Part model, mm, in its own coordinate system. Round coordinates to 2 decimals unless told otherwise and drop trailing zeros. Write each loop counter-clockwise with the first axis right and the second up, starting at its lowest first coordinate (ties: lowest second). Pieces come first, ordered by that corner, then holes.
1) Saw through at A-A on x = 129. Write the cut outline in (y, z), and give its area (3 significant figures).
2) Drill centre lines: L1, parallel to X at y = -22, z = 7; L2, parallel to X at y = 15, z = 6; L3, parallel to Y at x = 233.5, z = 3.5. Where is each one in solid material? Low to high.
3) Flat gauge pins, fed straight in: pin 1 (16 mm diameter, centred on x = 60.5, z = 14, fed in from +Y); pin 2 (5 mm diameter, centred on x = 95, y = -11, fed in from -Z); pin 3 (2.5 mm diameter, centred on x = -59.5, z = 6.5, fed in from -Y). Where does each tip first touch, or does it go through?
```python
from build123d import *

# Parameters (mm, degrees)
SKETCH1_R           = 10
BOSS_EXTRUDE1_DEPTH = 20
BOSS_EXTRUDE2_DEPTH = 20
SKETCH5_R           = 20
BOSS_EXTRUDE3_DEPTH = 5
CUT_EXTRUDE2_DEPTH  = 20
BOSS_EXTRUDE4_DEPTH = 20
CUT_EXTRUDE9_DEPTH  = 20
SKETCH13_R          = 10
CUT_EXTRUDE10_DEPTH = 20


with BuildPart() as part:
    # Sketch1 → Boss-Extrude1 (new body)
    with BuildSketch(Plane.XY):
        with BuildLine():
            Line((-71.370560529, 20), (333.629439471, 20))
            ThreePointArc((333.629439471, 20), (353.629439471, 0), (333.629439471, -20))
            Line((333.629439471, -20), (-71.370560529, -20))
            ThreePointArc((-71.370560529, -20), (-91.370560529, 0), (-71.370560529, 20))
        make_face()
        with Locations((-71.370560529, 0)):
            Circle(SKETCH1_R, mode=Mode.SUBTRACT)
        with Locations((333.629439471, 0)):
            Circle(SKETCH1_R, mode=Mode.SUBTRACT)
    extrude(amount=BOSS_EXTRUDE1_DEPTH)

    # Sketch2 → Boss-Extrude2 (add)
    with BuildSketch(Plane(origin=(0, 0, 0), x_dir=(-1, 0, 0), z_dir=(0, 0, -1))):
        with BuildLine():
            Line((71.370560529, -20), (71.370560529, -25))
            ThreePointArc((71.370560529, -25), (64.900084402, -24.148145657), (58.870560529, -21.650635095))
            Line((58.870560529, -21.650635095), (62.564306071, -17.956889553))
            ThreePointArc((62.564306071, -17.956889553), (66.850482602, -19.482527955), (71.370560529, -20))
        make_face()
    boss_extrude2 = extrude(amount=BOSS_EXTRUDE2_DEPTH)

    # Sketch5 → Boss-Extrude3 (add)
    with BuildSketch(Plane.XY.offset(15)):
        with Locations((-72.002203934, 0)):
            Circle(SKETCH5_R)
    extrude(amount=BOSS_EXTRUDE3_DEPTH)

    # Mirror1: Boss-Extrude2 across plane
    add(boss_extrude2.mirror(Plane.ZX))

    # Sketch7 → Cut-Extrude2 (cut)
    with BuildSketch(Plane(origin=(0, 0, -20), x_dir=(-1, 0, 0), z_dir=(0, 0, -1))):
        with BuildLine():
            Line((62.564306071, -17.956889553), (58.870560529, -21.650635095))
            ThreePointArc((58.870560529, -21.650635095), (64.900084402, -24.148145657), (71.370560529, -25))
            Line((71.370560529, -25), (71.370560529, -20))
            ThreePointArc((71.370560529, -20), (66.850482602, -19.482527955), (62.564306071, -17.956889553))
        make_face()
    extrude(amount=-CUT_EXTRUDE2_DEPTH, mode=Mode.SUBTRACT)

    # Sketch8 → Boss-Extrude4 (add)
    with BuildSketch(Plane.XY.offset(20)):
        Polygon((-85.646323907, 10.091030395), (-86.357789766, 21.677572637), (-81.372147128, 14.149030667), (-78.077875507, 25.280154567), (-75.967816914, 16.500449024), (-69.065145589, 25.833576761), (-70.085175248, 16.861669707), (-60.406668254, 23.271088335), (-64.433755534, 15.189124172), (-53.146783654, 17.901763211), (-59.695202395, 11.684546094), (-48.161141016, 10.373221242), (-56.441055274, 6.770639312), (-46.051082422, 1.593515699), (-55.06381234, 1.040093504), (-47.07111208, -7.378391356), (-55.729589416, -4.81590293), (-51.09819936, -15.460355519), (-58.35808396, -10.091030395), (-57.646618102, -21.677572637), (-62.63226074, -14.149030667), (-65.92653236, -25.280154567), (-68.036590954, -16.500449024), (-74.939262278, -25.833576761), (-73.91923262, -16.861669707), (-83.597739613, -23.271088335), (-79.570652334, -15.189124172), (-90.857624214, -17.901763211), (-84.309205472, -11.684546094), (-95.843266852, -10.373221242), (-87.563352593, -6.770639312), (-97.953325446, -1.593515699), (-88.940595528, -1.040093504), (-96.933295787, 7.378391356), (-88.274818452, 4.81590293), (-92.906208508, 15.460355519), align=None)
    extrude(amount=-BOSS_EXTRUDE4_DEPTH)

    # Sketch10 → Cut-Extrude9 (cut)
    with BuildSketch(Plane.XY.offset(20)):
        with BuildLine():
            Line((-86.6814877, -16.89809712), (-79.570652334, -15.189124172))
            Line((-79.570652334, -15.189124172), (-81.99592579, -20.056407098))
            ThreePointArc((-81.99592579, -20.056407098), (-84.438311294, -18.625022051), (-86.6814877, -16.89809712))
        make_face()
        with BuildLine():
            Line((-84.309205472, -11.684546094), (-88.22937615, -15.406444953))
            ThreePointArc((-88.22937615, -15.406444953), (-90.031123734, -13.238238107), (-91.547408648, -10.861623847))
            Line((-91.547408648, -10.861623847), (-84.309205472, -11.684546094))
        make_face()
        with BuildLine():
            Line((-87.563352593, -6.770639312), (-92.502393068, -8.919610595))
            ThreePointArc((-92.502393068, -8.919610595), (-93.457564825, -6.272216499), (-94.074540655, -3.526239548))
            Line((-94.074540655, -3.526239548), (-87.563352593, -6.770639312))
        make_face()
        with BuildLine():
            Line((-88.940595528, -1.040093504), (-94.312976138, -1.369981861))
            ThreePointArc((-94.312976138, -1.369981861), (-94.310669326, 1.447480522), (-93.956044653, 4.24253704))
            Line((-93.956044653, 4.24253704), (-88.940595528, -1.040093504))
        make_face()
        with BuildLine():
            Line((-88.274818452, 4.81590293), (-93.447669354, 6.346815359))
            ThreePointArc((-93.447669354, 6.346815359), (-92.482976347, 9.005039035), (-91.192268127, 11.521158668))
            Line((-91.192268127, 11.521158668), (-88.274818452, 4.81590293))
        make_face()
        with BuildLine():
            Line((-85.646323907, 10.091030395), (-90.005019716, 13.314670467))
            ThreePointArc((-90.005019716, 13.314670467), (-88.18159333, 15.49770898), (-86.097159024, 17.433083507))
            Line((-86.097159024, 17.433083507), (-85.646323907, 10.091030395))
        make_face()
        with BuildLine():
            Line((-81.372147128, 14.149030667), (-84.386387194, 18.700667134))
            ThreePointArc((-84.386387194, 18.700667134), (-81.909430889, 20.140547455), (-79.269488567, 21.253773582))
            Line((-79.269488567, 21.253773582), (-81.372147128, 14.149030667))
        make_face()
        with BuildLine():
            Line((-75.967816914, 16.500449024), (-77.253980818, 21.852025701))
            ThreePointArc((-77.253980818, 21.852025701), (-74.411990383, 22.361916972), (-71.52809096, 22.503419105))
            Line((-71.52809096, 22.503419105), (-75.967816914, 16.500449024))
        make_face()
        with BuildLine():
            Line((-70.085175248, 16.861669707), (-69.458212145, 22.376268852))
            ThreePointArc((-69.458212145, 22.376268852), (-66.592631783, 21.877869576), (-63.815360138, 21.013742934))
            Line((-63.815360138, 21.013742934), (-70.085175248, 16.861669707))
        make_face()
        with BuildLine():
            Line((-62.63226074, -14.149030667), (-59.556389162, -18.793733456))
            ThreePointArc((-59.556389162, -18.793733456), (-62.072733786, -20.218474816), (-64.751115176, -21.308498365))
            Line((-64.751115176, -21.308498365), (-62.63226074, -14.149030667))
        make_face()
        with BuildLine():
            Line((-68.036590954, -16.500449024), (-66.745286272, -21.873415875))
            ThreePointArc((-66.745286272, -21.873415875), (-69.575313157, -22.347843134), (-72.442716434, -22.457987779))
            Line((-72.442716434, -22.457987779), (-68.036590954, -16.500449024))
        make_face()
        with BuildLine():
            Line((-73.91923262, -16.861669707), (-74.538256817, -22.306440369))
            ThreePointArc((-74.538256817, -22.306440369), (-77.339471693, -21.79001562), (-80.052922922, -20.923596707))
            Line((-80.052922922, -20.923596707), (-73.91923262, -16.861669707))
        make_face()
    extrude(amount=-CUT_EXTRUDE9_DEPTH, mode=Mode.SUBTRACT)

    # Sketch13 → Cut-Extrude10 (cut)
    with BuildSketch(Plane(origin=(0, 0, 0), x_dir=(-1, 0, 0), z_dir=(0, 0, -1))):
        with Locations((71.370560529, 0)):
            Circle(SKETCH13_R)
    extrude(amount=-CUT_EXTRUDE10_DEPTH, mode=Mode.SUBTRACT)


solid = part.part
```
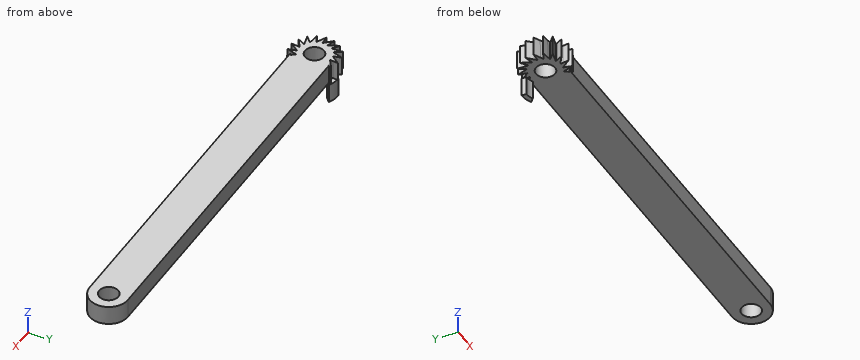
Completed:
1. outline: (-20, 0) - (20, 0) - (20, 20) - (-20, 20) - close
1. area: 800 mm2
2. L1: x = -82.96 to -81.68, -74.5 to -72.1, -66.71 to -64.96
2. L2: x = -92.71 to -92.28, -85.95 to -81.94, -81.12 to 346.86
2. L3: y = -20 to 20
3. pin 1: stops at y = 20
3. pin 2: stops at z = 0
3. pin 3: stops at y = -20.77
